Print and shaded views of the part. All mm, measured from the part's lowest x, y and z. A direction names the side the tool comes from. Round coordinates to 2 decimals unless told otherwise and drop trailing zeros. Write each loop counter-clockwise with the first axis right and the second up, starting at its lowest first coordinate (ties: lowest second). Pieces come first, ordered by that corner, then holes. Notation, with made-up numbers: (-11.5, 56.5) - (47.5, 56.5) arc R24 ccw to (47.5, 76.5) - close; hole circle Ø10 at (45, -33.75). An arc over 180 degrees is marked (long way). Put each result on its own line as item: value. Start each with the question number.
Item 1: 3-axis set-ups, long thin cutter, end or side, ignore diameter. For the marked faces 5, 6 and 7: which of +Z, -Z, +X, -X, +Y, -Y reach the whole face in a straight line?
Item 2: Cut at D-D (x = 23.5). Give the cut face in (y, z), and give its area (3 significant figures).
Item 3: Cut at B-B (x = 65). Give the cut face in (y, z).
Item 4: Drill centre lines: line 1 (Y direction, x = 65, z = 8.25); line 2 (X direction, y = 21.5, z = 24.5) (1 decimal); line 3 (X direction, y = 29, z = 24.5) (1 decimal). Where is each one in solid material? Low to high. Write a range as from..to.
Item 5: Pin check, flat tips, straight feed: pin 1 Ø6 at (y, z) = (39.5, 28.5) entering from +X; pin 2 Ø10 at (x, y) = (44, 7.5) entering from +Z; pin 3 Ø12 at (y, z) = (18.5, 12.5) entering from +X. Stop position of each tip, or through.
Item 6: Cut at C-C (z = 14). Give the cut face in (x, y), and give its area (3 significant figures).
Item 7: Mould opens along Y. For the marked faces 1, 2, 3 and 4 say: released by +Y, released by -Y, zero draft, split by the parting line, or undercut.
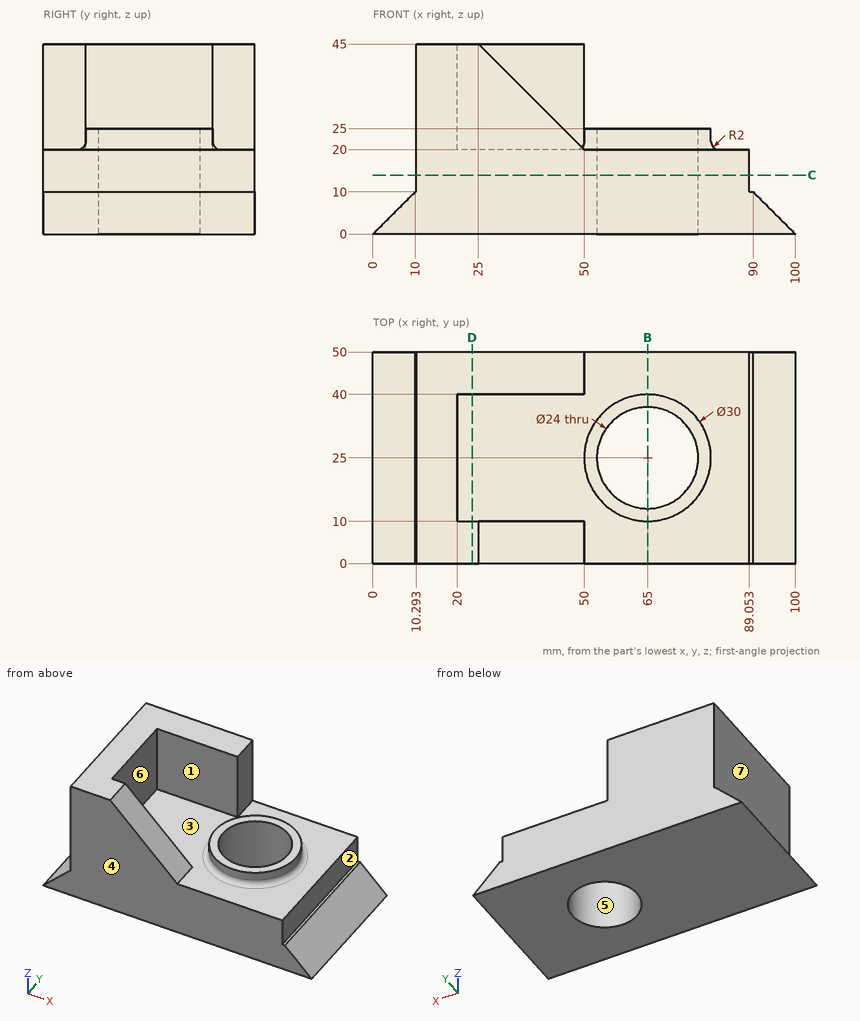
Output values:
1. face 5: +Z, -Z
1. face 6: +Z
1. face 7: +Z, -X, +Y, -Y
2. outline: (0, 0) - (50, 0) - (50, 45) - (40, 45) - (40, 20) - (10, 20) - (10, 45) - (0, 45) - close
2. area: 1,500 mm2
3. outline: (0, 0) - (13, 0) - (13, 25) - (10, 25) - (10, 22) arc R2 cw to (8, 20) - (0, 20) - close; (37, 0) - (50, 0) - (50, 20) - (42, 20) arc R2 cw to (40, 22) - (40, 25) - (37, 25) - close
4. line 1: 0..13, 37..50
4. line 2: 10.3..20, 50.4..53.5, 76.5..79.6
4. line 3: 10.3..20, 50.5..53.7, 76.3..79.5
5. pin 1: x = 50
5. pin 2: z = 31
5. pin 3: x = 93.5
6. outline: (10.29, 0) - (89.05, 0) - (89.05, 50) - (10.29, 50) - close; hole circle Ø24 at (65, 25)
6. area: 3,490 mm2
7. face 1: undercut
7. face 2: zero draft
7. face 3: undercut
7. face 4: released by -Y
